Geometry: see drawing. Coordinates: mm, zero at the bounding-box minimum. Give positions to 0.01 mm unless a question says otherwise; leave off trailing zeros. Order: outer loops, then holes, each group sorted by start corner. A loop starts at its lowest first (then second) coordinate and runs counter-clockwise, first axis right, second up. Notation, with made-up numbers: (-38, 29) -> (-19, 29) arc R32 cw to (-19, 63) -> close; hole circle Ø9 at (75, -9). An arc over 180 degrees is marked (long way). One line per item, written item: value. Start each with the question number.
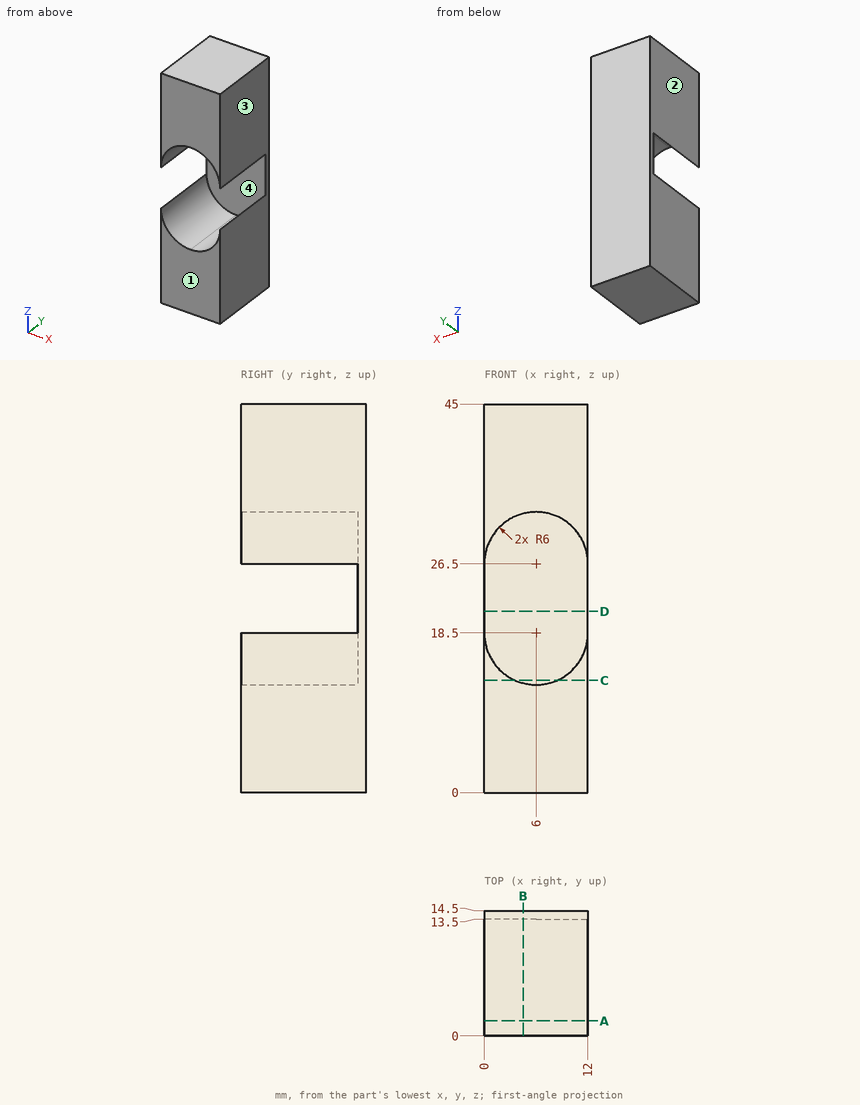
1. Cut plane A-A, the plane y = 1.75. Return loops of the section in (x, z).
2. Draft query along X for the marked faces 1, 2, 3 and 4. Return one class per face: pulls with the +X half, pulls with the -X half, needs draft (parallel to the pull), parting line crosses it, or undercut.
3. Cut plane B-B, the plane x = 4.5. Return loops of the section in (y, z), then the cut area to 3 significant figures.
4. Material intervals for L1, parallel to Z at x = 3, y = 4; L2, parallel to Y at x = 7.25, z = 14.5; L3, parallel to Z at x = 7.75, y = 9, sorted ascending. Write a range as [from, to].
5. Cut plane D-D, the plane z = 21. Return loops of the section in (x, y), then the cut area to 3 significant figures.
6. Cut plane C-C, the plane z = 13. Return loops of the section in (x, y), then the cut area to 3 significant figures.
Answers follow:
1. outline: (0, 0) -> (12, 0) -> (12, 18.5) arc R6 cw to (0, 18.5) -> close; (0, 26.5) arc R6 cw to (12, 26.5) -> (12, 45) -> (0, 45) -> close
2. face 1: needs draft
2. face 2: pulls with the -X half
2. face 3: pulls with the +X half
2. face 4: undercut
3. outline: (0, 0) -> (14.5, 0) -> (14.5, 45) -> (0, 45) -> (0, 32.31) -> (13.5, 32.31) -> (13.5, 12.69) -> (0, 12.69) -> close
3. area: 388 mm²
4. L1: z = [0, 13.3], [31.7, 45]
4. L2: y = [13.5, 14.5]
4. L3: z = [0, 12.76], [32.24, 45]
5. outline: (0, 13.5) -> (12, 13.5) -> (12, 14.5) -> (0, 14.5) -> close
5. area: 12.0 mm²
6. outline: (0, 0) -> (3.6, 0) -> (3.6, 13.5) -> (8.4, 13.5) -> (8.4, 0) -> (12, 0) -> (12, 14.5) -> (0, 14.5) -> close
6. area: 109 mm²
